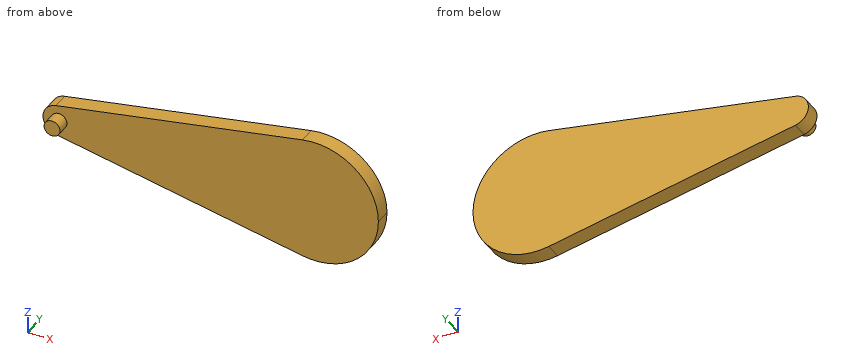
from build123d import *

# Parameters (mm, degrees)
F1_DEPTH = 3.175
F2_R     = 1.5875
F3_DEPTH = 2.54


with BuildPart() as f1:
    # F0 (on Front) → F1 (new body)
    with BuildSketch(Plane.XZ):
        with BuildLine():
            ThreePointArc((-0.595313, -3.11869), (2.023673, -2.446502), (3.175, 0))
            ThreePointArc((3.175, 0), (2.023673, 2.446502), (-0.595313, 3.11869))
            ThreePointArc((-0.595313, 3.11869), (-3.175, 0), (-0.595313, -3.11869))
        make_face()
        with BuildLine():
            ThreePointArc((-0.595313, 3.11869), (2.023673, 2.446502), (3.175, 0))
            ThreePointArc((3.175, 0), (2.023673, -2.446502), (-0.595313, -3.11869))
            Line((-0.595313, -3.11869), (48.41875, -12.47476))
            ThreePointArc((48.41875, -12.47476), (38.1, 0), (48.41875, 12.47476))
            Line((48.41875, 12.47476), (-0.595313, 3.11869))
        make_face()
        with BuildLine():
            ThreePointArc((63.5, 0), (58.894693, 9.786007), (48.41875, 12.47476))
            ThreePointArc((48.41875, 12.47476), (38.1, 0), (48.41875, -12.47476))
            ThreePointArc((48.41875, -12.47476), (58.894693, -9.786007), (63.5, 0))
        make_face()
    extrude(amount=F1_DEPTH)

    # F2 (on face) → F3 (join)
    with BuildSketch(Plane.XZ.offset(3.175)):
        Circle(F2_R)
    extrude(amount=F3_DEPTH)


solid = f1.part
Read the model definition and answer for the solid it produces. Units are mm, in the model's axes. Round coordinates to 2 decimals unless told otherwise and drop trailing zeros. Order: outer loops, then holes, each group sorted by start corner. A loop starts at its lowest first (then second) coordinate and runs counter-clockwise, first axis right, second up.
1) Straight lines are drawn through the part: L1, parallel to Y at x = 34.5, z = 8 (3 decimals); L2, parallel to Z at x = 47, y = -0.3; L3, parallel to Z at x = 47.5, y = -1.35. For each, find the intervals that lie inside material, in ascending order.
2) The part is cut by section D-D on y = -4.45. Write down the section's boundary in (x, z) (1 decimal).
3) The part is cut by section A-A on y = -1.65. Write down the section's boundary in (x, z) (3 decimals), plus the area to 3 significant figures.
4) Flat-ended cylindrical pins translate along their axes: pin 1 (1.5 mm diameter, centred on x = 56.5, z = -2.5, fed in from -Y) (3 decimals); pin 2 (1.5 mm diameter, centred on y = -4, z = 2.5, fed in from +X); pin 3 (3 mm diameter, centred on x = 4, y = -1, fed in from +Z). Find the tip coordinate at first contact, or state that the pin passes through.
5) The part is cut by section B-B on x = 0. Write down the section's boundary in (y, z) (1 decimal), plus the area to 3 significant figures.
6) The part is cut by section C-C on z = -6. Write down the section's boundary in (x, y) (3 decimals), plus the area to 3 significant figures.
Resolved:
1. L1: y = -3.175 to 0
1. L2: z = -12.2 to 12.2
1. L3: z = -12.3 to 12.3
2. outline: circle Ø3.2 at (0, 0)
3. outline: (-0.595, -3.119) - (48.419, -12.475) arc R12.7 ccw to (63.5, 0) arc R12.7 ccw to (48.419, 12.475) - (-0.595, 3.119) arc R3.175 ccw to start
3. area: 1,090 mm2
4. pin 1: stops at y = -3.175
4. pin 2: passes through
4. pin 3: stops at z = 4.28
5. outline: (-5.7, -1.6) - (-3.2, -1.6) - (-3.2, -3.2) - (0, -3.2) - (0, 3.2) - (-3.2, 3.2) - (-3.2, 1.6) - (-5.7, 1.6) - close
5. area: 28.6 mm2
6. outline: (14.499, -3.175) - (61.993, -3.175) - (61.993, 0) - (14.499, 0) - close
6. area: 151 mm2
